Autodesk Inventor part; units mm, degrees
ref_plane "YZ Plane" through (0, 0, 0) normal (1, 0, 0) x (0, 1, 0)
ref_plane "XZ Plane" through (0, 0, 0) normal (0, 1, 0) x (-1, 0, 0)
ref_plane "XY Plane" through (0, 0, 0) normal (0, 0, 1) x (1, 0, 0)
sketch "Sketch1" plane through (0, 0, 0) normal (0, 1, 0) x (-1, 0, 0)
  circle A0 centre (0, 0) radius 1.5
  circle A1 centre (0, 0) radius 2
  dimension "d0" = 3
  dimension "d1" = 4
extrude "Extrusion1" add sketch "Sketch1" along normal blind 2
sketch "Sketch2" plane through (0, 2, 0) normal (0, 1, 0) x (1, 0, 0)
  line L0 (-1.9117, -0.1) -> (-2.7237, -0.1) construction
  line L1 (-2.7237, -0.1) -> (-2.7237, 0.1) construction
  line L2 (-2.7237, 0.1) -> (-1.9117, 0.1) construction
  line L3 (-1.9117, 0.1) -> (-1.9117, -0.1) construction
  line L4 (-1.9117, 0) -> (-1.9117, 0.35) construction
  line L5 (-1.9117, 0) -> (-1.5617, 0) construction
  line L6 (-1.9117, 0.35) -> (-1.9117, -0.35) construction
  line L7 (-1.9117, 0.1) -> (-2.9669, 0.1) construction
  line L8 (-2.9669, 0.1) -> (-2.9669, -0.1) construction
  line L9 (-2.9669, -0.1) -> (-1.9117, -0.1) construction
  line L10 (-1.9117, -0.1) -> (-1.9117, 0.1) construction
  arc A0 (-2.9669, -0.1) -> (-1.9117, -0.35) centre (-2.1069, 1.1781) ccw construction
  arc A1 (-2.9669, -0.1) -> (-1.9117, -0.35) centre (-2.1069, 1.1781) ccw
  arc A2 (-1.9117, 0.35) -> (-2.9669, 0.1) centre (-2.1068, -1.1786) ccw
  line L11 (-2.9669, -0.1) -> (-2.9669, 0.1)
  line L12 (-1.9117, -0.35) -> (-1.9117, 0.35)
  point P0 (0, 0)
  dimension "d4" = 0.2
  dimension "d5" = 0.35
  dimension "d6" = 90
  dimension "d7" = 0.7
  dimension "d8" = 1.541
extrude "Extrusion2" add sketch "Sketch2" against normal blind 2
pattern_circular "Circular Pattern1" count 8 over 360 about axis through (0, 0, 0) along (0, 1, 0) of "Extrusion2"
properties part number "mtv_gear8_1-13"
Check sheet for the modelled part. Datum: model origin and axes. Units: mm. A direction names the side the tool comes from. Coordinates: 2 decimals unless noted, no trailing zeros. Write each loop counter-clockwise with the first axis right and the second up, starting at its lowest first coordinate (ties: lowest second). Pieces come first, ordered by that corner, then holes. Notation, with made-up numbers: M 55.5,33 L 104.5,33 A8 ccw 104.5,47 Z; hole C -1,65.5 d8. An arc over 180 degrees is marked long. Use one line per item in the form item = value.
Item 1: Set-up check for faces 4 (the face through (-1.979, 1.014, 1.532)), 5 (the face through (1.545, 1.014, -1.986)), 6 (the face through (0, 0, 2)), 7 (the face through (1.532, 1.014, 1.979)): record each of +Z, -Z, +X, -X, +Y, -Y from which the full face is reachable in a straight line by a thin tool's end or side.
Answer below:
face_4 = -X, +Y, -Y
face_5 = -Z, +Y, -Y
face_6 = +Z, -Z, +X, -X, -Y
face_7 = +Z, +Y, -Y
Item 2: Sectioned sample at D-D, the plane x = 1.75. Record the cut outline in (y, z).
Answer below:
outline = M 0,-2.09 L 2,-2.09 L 2,-1.24 L 0,-1.24 Z; M 0,-0.97 L 2,-0.97 L 2,0.97 L 0,0.97 Z; M 0,1.24 L 2,1.24 L 2,2.09 L 0,2.09 Z
Item 3: Sectioned sample at C-C, the plane z = 0. Record the cut outline in (x, y), and give its area (3 significant figures).
Answer below:
outline = M -2.97,0 L -1.5,0 L -1.5,2 L -2.97,2 Z; M 1.5,0 L 2.97,0 L 2.97,2 L 1.5,2 Z
area = 5.87 mm^2
Item 4: Release check for a two-part mould opening along X. For faces 1 (the face through (1.986, 1.014, 1.545)), 2 (the face through (0, 2, 2)), 3 (the face through (-1.545, 1.014, 1.986)) record: pulls with the +X half, pulls with the -X half, needs draft (parallel to the pull), parting line crosses it, or undercut.
Answer below:
face_1 = pulls with the +X half
face_2 = needs draft
face_3 = undercut
Item 5: Material ranges on L1, parallel to Z at x = 0, y = 1; L2, parallel to X at y = 1.45, z = 1.8; L3, parallel to Z at x = 0.9, y = 1.05, recorded low to high. Write a range as from..to.
Answer below:
L1 = -2.97..-1.5, 1.5..2.97
L2 = -2.11..-1.29, -0.87..0.87, 1.29..2.11
L3 = -1.79..-1.2, 1.2..1.79
Item 6: Sectioned sample at B-B, the plane x = 0. Record the cut outline in (y, z), and give its area (3 significant figures).
Answer below:
outline = M 0,-2.97 L 2,-2.97 L 2,-1.5 L 0,-1.5 Z; M 0,1.5 L 2,1.5 L 2,2.97 L 0,2.97 Z
area = 5.87 mm^2
